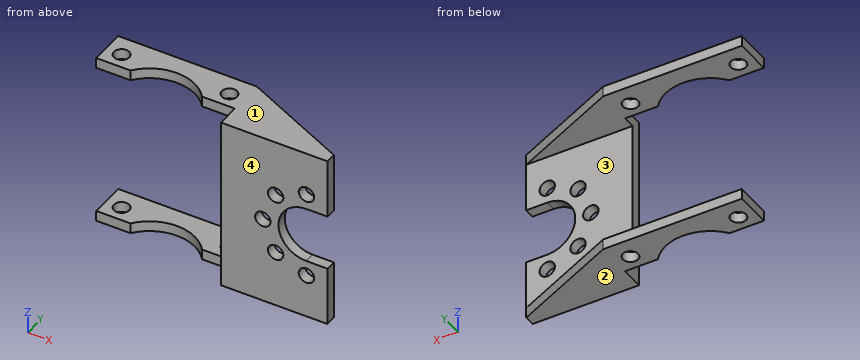
from build123d import *

# Parameters (mm, degrees)
F0_W      = 20
F0_H      = 1.5
F1_DEPTH  = 12.5
F2_W      = 20
F2_H      = 1.5
F3_DEPTH  = 8.5
F4_R      = 1.1
F5_DEPTH  = 1.5
F8_DEPTH  = 15
F9_R      = 1.1
F9_W      = 19.8
F9_H      = 25
F10_DEPTH = 3.3
F12_DEPTH = 25.001


with BuildPart() as f1:
    # F0 (on Top) → F1 (new body)
    with BuildSketch(Plane.XY):
        Rectangle(F0_W, F0_H)
    extrude(amount=F1_DEPTH)

    # F2 (on face) → F3 (join)
    with BuildSketch(Plane(origin=(0, 0.75, 0), x_dir=(-1, 0, 0), z_dir=(0, 1, 0))):
        with Locations((0, 11.75)):
            Rectangle(F2_W, F2_H)
    extrude(amount=F3_DEPTH)

    # F4 (on face) → F5 (cut, through all)
    with BuildSketch(Plane.XY.offset(12.5)):
        with Locations((-7.7, 4.75)):
            Circle(F4_R)
        with Locations((7.7, 4.75)):
            Circle(F4_R)
    extrude(amount=-F5_DEPTH, mode=Mode.SUBTRACT)

    # F6: F1 across plane


with BuildPart() as f1_1:
    add(f1.part)
    add(f1.part.mirror(Plane.XY))

    # F7 (on face) → F8 (join)
    with BuildSketch(Plane.YZ.offset(10)):
        Polygon((5.85, -12.5), (9.25, -12.5), (9.25, -11), (5.85, -11), (3.65, -11), (0.75, -11), (0.75, 11), (3.65, 11), (5.85, 11), (9.25, 11), (9.25, 12.5), (5.85, 12.5), (3.65, 12.5), (-0.75, 12.5), (-0.75, -12.5), (3.65, -12.5), align=None)
    extrude(amount=F8_DEPTH)

    # F9 (on face) → F10 (cut)
    with BuildSketch(Plane.XZ.offset(0.75)):
        with BuildLine():
            Line((25, 4), (22, 4))
            ThreePointArc((22, 4), (18, 0), (22, -4))
            Line((22, -4), (25, -4))
            Line((25, -4), (25, 4))
        make_face()
        with Locations((17.6, -4.4)):
            Circle(F9_R)
        with Locations((22, -6.2225396744)):
            Circle(F9_R)
        with Locations((22, 6.2225396744)):
            Circle(F9_R)
        with Locations((17.6, 4.4)):
            Circle(F9_R)
        with Locations((15.7774603256, 0)):
            Circle(F9_R)
        with Locations((-0.1, 0)):
            Rectangle(F9_W, F9_H)
    extrude(amount=-F10_DEPTH, mode=Mode.SUBTRACT)

    # F11 (on face) → F12 (cut, through all)
    with BuildSketch(Plane.XY.offset(12.5)):
        with BuildLine():
            Line((-5.123475383, 2.55), (5.123475383, 2.55))
            ThreePointArc((5.123475383, 2.55), (0, 5.05), (-5.123475383, 2.55))
        make_face()
        Polygon((-10, 9.25), (-10, 7.75), (9.8, 7.75), (25, 0.75), (25, 9.25), align=None)
    extrude(amount=-F12_DEPTH, mode=Mode.SUBTRACT)


solid = f1_1.part
Read the model definition and answer for the solid it produces. Units are mm, in the model's axes. Face numbers are marked on the shaded views. Give positions to 0.01 mm unless a question says otherwise; leave off trailing zeros. Write each loop counter-clockwise with the first axis right and the second up, starting at its lowest first coordinate (ties: lowest second). Pieces come first, ordered by that corner, then holes. Notation, with made-up numbers: (56, 23.25) - (93, 23.25) arc R18 cw to (93, 40.25) - close; hole circle Ø10 at (-12, 74.25). An arc over 180 degrees is marked (long way). Return JSON: item names as keys, results as strings.
Q1. A cutting plane is placed at C-C, the plane y = 6.75. Determine the outline of the cut face in (x, z), and give its area (3 significant figures).
Reply:
{"outline": "(-10, -12.5) - (11.97, -12.5) - (11.97, -11) - (-10, -11) - close; (-10, 11) - (11.97, 11) - (11.97, 12.5) - (-10, 12.5) - close", "area": "65.9 mm²"}
Q2. A cutting plane is placed at D-D, the plane x = 20. Determine the outline of the cut face in (y, z).
Reply:
{"outline": "(-0.75, -12.5) - (3.05, -12.5) - (3.05, -11) - (0.75, -11) - (0.75, -3.46) - (-0.75, -3.46) - close; (-0.75, 3.46) - (0.75, 3.46) - (0.75, 11) - (3.05, 11) - (3.05, 12.5) - (-0.75, 12.5) - close"}
Q3. For a pull along Z with two mould halves and no side action, classify the marked faces 1, 2, 3 and 4 as released by +Z, released by -Z, zero draft, split by the parting line, or undercut.
Reply:
{"face 1": "released by +Z", "face 2": "released by -Z", "face 3": "undercut", "face 4": "zero draft"}
Q4. Given P1, Ø3.5, axis at y = 0, z = -4.5, coming from the -X side; P2, Ø1.5, axis at x = 12, z = 5.5, coming from the +Y side; P3, Ø1.2, axis at x = 8, z = -11.5, coming from the -Y side, each flat-ended and moving along its own axis, determine where each tip first touches the part or whether it passes through.
Reply:
{"P1": "x = 9.8", "P2": "y = 0.75", "P3": "y = 2.55"}
Q5. A cutting plane is placed at A-A, the plane z = 0. Determine the outline of the cut face in (x, y), and give its area (3 significant figures).
Reply:
{"outline": "(9.8, -0.75) - (14.68, -0.75) - (14.68, 0.75) - (9.8, 0.75) - close; (16.88, -0.75) - (18, -0.75) - (18, 0.75) - (16.88, 0.75) - close", "area": "9.00 mm²"}
Q6. A cutting plane is placed at B-B, the plane x = 7.7. Determine the outline of the cut face in (y, z), and give its area (3 significant figures).
Reply:
{"outline": "(2.55, -12.5) - (3.65, -12.5) - (3.65, -11) - (2.55, -11) - close; (2.55, 11) - (3.65, 11) - (3.65, 12.5) - (2.55, 12.5) - close; (5.85, -12.5) - (7.75, -12.5) - (7.75, -11) - (5.85, -11) - close; (5.85, 11) - (7.75, 11) - (7.75, 12.5) - (5.85, 12.5) - close", "area": "9.00 mm²"}
Q7. Consider line 1 along Z through (x, y) = (17.6, -0.3); line 2 along Z through (x, y) = (22, 0); line 3 along Z through (x, y) = (18, 2). Determine where each line is inside the solid, lowest interval first. Write a range as [from, to].
Reply:
{"line 1": "[-12.5, -5.5], [-3.3, 3.3], [5.5, 12.5]", "line 2": "[-12.5, -7.32], [-5.12, -4], [4, 5.12], [7.32, 12.5]", "line 3": "[-12.5, -11], [11, 12.5]"}
